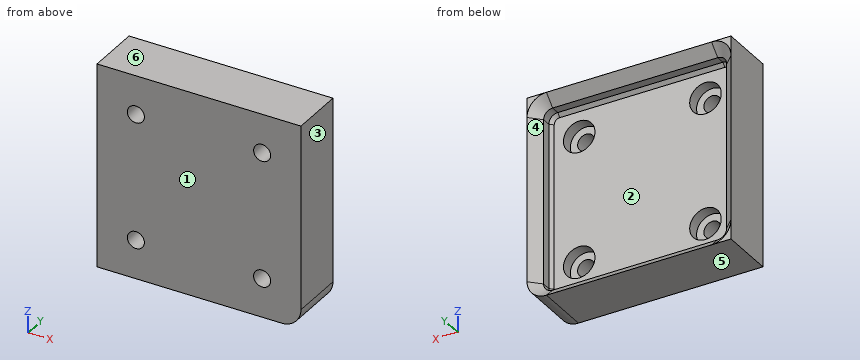
Autodesk Inventor part; units mm, degrees
ref_plane "YZ Plane" through (0, 0, 0) normal (1, 0, 0) x (0, 1, 0)
ref_plane "XZ Plane" through (0, 0, 0) normal (0, 1, 0) x (-1, 0, 0)
ref_plane "XY Plane" through (0, 0, 0) normal (0, 0, 1) x (1, 0, 0)
sketch "Sketch1" plane through (0, 0, 0) normal (0, 1, 0) x (-1, 0, 0)
  line L0 (0, -42) -> (-38, -42)
  line L1 (-42, -38) -> (-42, 0)
  line L2 (-42, 0) -> (0, 0)
  line L3 (0, 0) -> (0, -42)
  arc A0 (-42, -38) -> (-38, -42) centre (-38, -38) ccw
  point P0 (-42, -42)
  dimension "d0" = 42
  dimension "d1" = 42
  dimension "d31" = 4
extrude "square-base" add sketch "Sketch1" along normal blind 4.65
sketch "Sketch2" plane through (0, 4.65, 0) normal (0, 1, 0) x (1, 0, 0)
  line L0 (4, 39.15) -> (38, 39.15)
  line L1 (39.15, 38) -> (39.15, 4)
  line L2 (38, 2.85) -> (4, 2.85)
  line L3 (2.85, 4) -> (2.85, 38)
  line L4 (38, 42) -> (0, 42)
  line L5 (0, 42) -> (0, 0)
  line L6 (42, 0) -> (42, 38)
  line L7 (0, 0) -> (42, 0)
  arc A0 (39.15, 38) -> (38, 39.15) centre (38, 38) ccw
  arc A1 (38, 2.85) -> (39.15, 4) centre (38, 4) ccw
  arc A2 (2.85, 4) -> (4, 2.85) centre (4, 4) ccw
  arc A3 (4, 39.15) -> (2.85, 38) centre (4, 38) ccw
  point P0 (2.85, 39.15)
  point P1 (39.15, 2.85)
  point P2 (39.15, 39.15)
  point P3 (2.85, 2.85)
  point P4 (42, 42)
  dimension "d4" = 2.85
  dimension "d5" = 2.85
  dimension "d6" = 2.85
  dimension "d7" = 2.85
  dimension "d29" = 1.15
extrude "Extrusion2" cut sketch "Sketch2" against normal through all
sketch "Sketch3" plane through (0, 4.65, 0) normal (0, 1, 0) x (1, 0, 0)
  line L0 (38, 2.15) -> (4, 2.15)
  line L1 (2.15, 4) -> (2.15, 38)
  line L2 (4, 39.85) -> (38, 39.85)
  line L3 (39.85, 38) -> (39.85, 4)
  line L4 (0, 42) -> (0, 0)
  line L5 (38, 2.85) -> (4, 2.85)
  line L6 (42, 0) -> (42, 38)
  line L7 (38, 42) -> (0, 42)
  line L8 (0, 0) -> (42, 0)
  line L9 (39.15, 38) -> (39.15, 4)
  line L10 (2.85, 4) -> (2.85, 38)
  line L11 (4, 39.15) -> (38, 39.15)
  arc A0 (39.85, 38) -> (38, 39.85) centre (38, 38) ccw
  arc A1 (38, 2.15) -> (39.85, 4) centre (38, 4) ccw
  arc A2 (2.15, 4) -> (4, 2.15) centre (4, 4) ccw
  arc A3 (4, 39.85) -> (2.15, 38) centre (4, 38) ccw
  point P0 (39.85, 2.15)
  point P1 (2.15, 39.85)
  point P2 (2.15, 2.15)
  point P3 (39.85, 39.85)
  point P4 (39.15, 2.85)
  point P5 (2.85, 2.85)
  point P6 (42, 42)
  point P7 (39.15, 39.15)
  point P8 (2.85, 39.15)
  dimension "d10" = 2.15
  dimension "d12" = 2.15
  dimension "d13" = 2.15
  dimension "d14" = 2.15
  dimension "d30" = 1.85
extrude "Extrusion3" cut sketch "Sketch3" against normal blind 3.95
chamfer "Chamfer2" distance 0.7 angle 45 4 edges at (39.15, 0.7, -21) (21, 0.7, -2.85) (2.85, 0.7, -21) (21, 0.7, -39.15)
chamfer "Chamfer1" distance 2.15 angle 45 8 edges at (39.85, 4.65, -21) (39.3081, 4.65, -2.6919) (21, 4.65, -2.15) (2.6919, 4.65, -2.6919) (2.15, 4.65, -21) (2.6919, 4.65, -39.3081) (21, 4.65, -39.85) (39.3081, 4.65, -39.3081)
sketch "Sketch5" plane through (0, 0, 0) normal (0, -1, 0) x (1, 0, 0)
  arc A0 (38, -39.15) -> (39.15, -38) centre (38, -38) ccw
  line L0 (38, -39.15) -> (4, -39.15)
  arc A1 (2.85, -38) -> (4, -39.15) centre (4, -38) ccw
  line L1 (2.85, -38) -> (2.85, -4)
  arc A2 (4, -2.85) -> (2.85, -4) centre (4, -4) ccw
  line L2 (4, -2.85) -> (38, -2.85)
  arc A3 (39.15, -4) -> (38, -2.85) centre (38, -4) ccw
  line L3 (39.15, -4) -> (39.15, -38)
  line L4 (38, -42) -> (0, -42)
  arc A4 (38, -42) -> (42, -38) centre (38, -38) ccw
  line L5 (42, 0) -> (42, -38)
  line L6 (0, 0) -> (42, 0)
  line L7 (0, -42) -> (0, 0)
extrude "weighted-base" add sketch "Sketch5" along normal blind 6.5 contours L0 A1 L1 A2 L2 A3 L3 A0 | L4 L7 L6 L5 A4
sketch "Sketch6" plane through (0, 0, 0) normal (0, 1, 0) x (1, 0, 0)
  circle A0 centre (34, 8) radius 3.25
  circle A1 centre (8, 8) radius 3.25
  circle A2 centre (34, 34) radius 3.25
  circle A3 centre (8, 34) radius 3.25
  line L0 (4, 0) -> (38, 0)
  line L1 (42, 4) -> (42, 38)
  line L2 (38, 42) -> (4, 42)
  line L3 (0, 38) -> (0, 4)
  point P0 (0, 0)
  dimension "d34" = 6.5
  dimension "d35" = 8
  dimension "d36" = 8
  dimension "d37" = 8
  dimension "d38" = 8
extrude "Extrusion5" cut sketch "Sketch6" against normal blind 2.4
sketch "Sketch7" plane through (34, -2.4, -8) normal (0, 1, 0) x (1, 0, 0)
  circle A0 centre (0, 0) radius 1.75
  circle A1 centre (-26, 0) radius 1.75
  circle A2 centre (-26, 26) radius 1.75
  circle A3 centre (0, 26) radius 1.75
  circle A4 centre (0, 0) radius 3.25
  circle A5 centre (-26, 0) radius 3.25
  circle A6 centre (-26, 26) radius 3.25
  circle A7 centre (0, 26) radius 3.25
  point P0 (-34, -8)
  dimension "d41" = 3.5
extrude "Extrusion6" cut sketch "Sketch7" against normal through all contours A0 | A1 | A2 | A3
equation "\"d1\" = d0"
equation "\"d5\" = d4"
equation "\"d6\" = d4"
equation "\"d7\" = d4"
equation "\"d12\" = d10"
equation "\"d13\" = d10"
equation "\"d14\" = d10"
equation "\"d36\" = d35"
equation "\"d37\" = d35"
equation "\"d38\" = d35"
properties part number "base-plate-weighted"
Read the model definition and answer for the solid it produces. Units are mm, in the model's axes. Face numbers are marked on the shaded views. A direction names the side the tool comes from. Give positions to 0.01 mm unless a question says otherwise; leave off trailing zeros. Write each loop counter-clockwise with the first axis right and the second up, starting at its lowest first coordinate (ties: lowest second). Pieces come first, ordered by that corner, then holes. Notation, with made-up numbers: M 30,-13 L 49,-13 A26 cw 49,6 Z; hole C 26.5,59 d2. An arc over 180 degrees is marked long. One line per item, written item: value. Start each with the question number.
(1) Find section C-C (y = -3). Determine the outline of the cut face in (x, z).
(2) Flat-ended cylindrical pins translate along their axes: pin 1 Ø7 at (x, z) = (33.5, -33) entering from +Y; pin 2 Ø2 at (x, z) = (7.5, -35.5) entering from +Y. Find the tip coordinate at first contact, or state that the pin passes through.
(3) Find the intervals of material crossed by line 1 (X direction, y = -0.7, z = -34); line 2 (Z direction, x = 34, y = -5.3); line 3 (Z direction, x = 34, y = -0.75), in increasing order.
(4) Determine the mould class of the marked faces 3, 4, 5 and 6 for opening direction Z: pulls with the +Z half, pulls with the -Z half, needs draft (parallel to the pull), parting line crosses it, or undercut.
(5) Find section A-A (z = -34). Give the number of separate pieces and of enclosed holes in the cut face, plus the area to 3 significant figures.
(6) A tool of negligible diameter and unlimited length cuts with its end or side. For the marked faces 1 and 2, from which of +Z, -Z, +X, -X, +Y, -Y can it reach the whole face along a straight path? Write none if from no direction.
Results below:
1. outline: M 0,-42 L 38,-42 A4 ccw 42,-38 L 42,0 L 0,0 Z; hole C 8,-34 d3.5; hole C 8,-8 d3.5; hole C 34,-34 d3.5; hole C 34,-8 d3.5
2. pin 1: stops at y = 0
2. pin 2: stops at y = -2.4
3. line 1: x = 0 to 4.75, 11.25 to 30.75, 37.25 to 42
3. line 2: z = -42 to -35.75, -32.25 to -9.75, -6.25 to 0
3. line 3: z = -42 to -37.25, -30.75 to -11.25, -4.75 to 0
4. face 3: needs draft
4. face 4: undercut
4. face 5: pulls with the -Z half
4. face 6: pulls with the +Z half
5. separate pieces: 3
5. enclosed holes: 0
5. area: 229 mm^2
6. face 1: +Z, -Z, +X, -X, -Y
6. face 2: +Y
